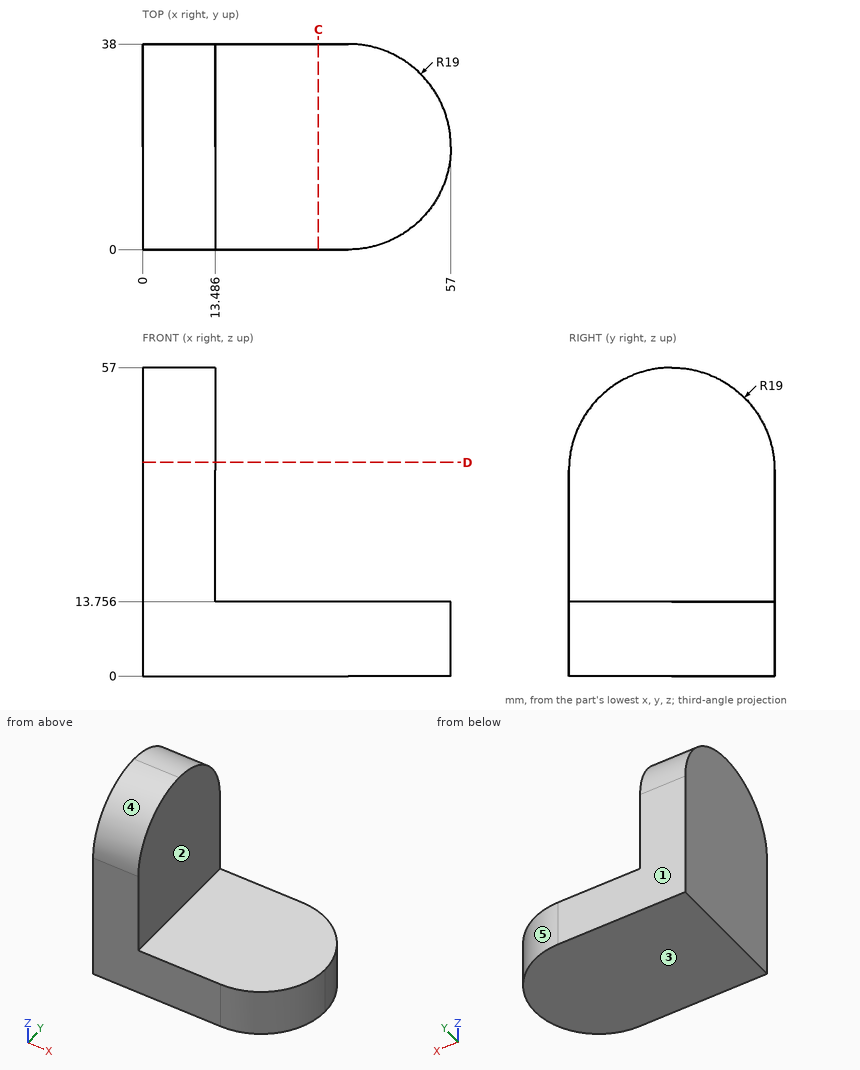
Geometry check sheet. Reference: drawing and pictorial views, mm from the part's lowest x, y, z. A direction names the side the tool comes from. Coordinates: 2 decimals unless noted, no trailing zeros. Order: outer loops, then holes, each group sorted by start corner. A loop starts at its lowest first (then second) coordinate and runs counter-clockwise, first axis right, second up. Notation, with made-up numbers: M 33,67.25 L 80,67.25 A26 cw 80,97.25 Z; hole C -11,57 d7. An arc over 180 degrees is marked long. Write each question's results on one line, items separated by ' | '. Start each with the question number.
1. Mould release check, pull along Z, two halves, no side actions. Record for the marked faces 3, 4 and 5: +Z half, -Z half, draft (parallel to the pull), parting line (faces both ways), or undercut.
2. Material ranges on probe 1 along X at (y, z) = (25, 49) (1 decimal); probe 2 along Z at (x, y) = (47, 27) (1 decimal); probe 3 along X at (y, z) = (18.5, 9), recorded low to high.
3. Go/stop test with flat-tipped pins: P1, Ø10, axis at y = 17.5, z = 29.5, coming from the +X side; P2, Ø3, axis at y = 25.5, z = 41, coming from the -X side; P3, Ø12, axis at x = 44.5, z = 12.5, coming from the +Y side; P4, Ø10, axis at x = 30.5, y = 5.5, coming from the +Z side. Record where each tip stops, or that it passes through.
4. Cross-section at D-D on z = 39.5. Record the cut outline in (x, y) (1 decimal), and give its area (3 significant figures).
5. Access from +Z, -Z, +X, -X, +Y, -Y to the whole of each face (thin tool, end or side, straight path). Record for the marked faces 1 and 2.
6. Cross-section at C-C on x = 32.5. Record the cut outline in (y, z) (1 decimal).
Checks:
1) face 3: -Z half | face 4: +Z half | face 5: draft
2) probe 1: x = 0 to 13.5 | probe 2: z = 0 to 13.8 | probe 3: x = 0 to 56.99
3) P1: stops at x = 13.49 | P2: stops at x = 0 | P3: stops at y = 37.99 | P4: stops at z = 13.76
4) outline: M 0,0.1 L 13.5,0.1 L 13.5,37.9 L 0,37.9 Z | area: 511 mm²
5) face 1: +Z, -Z, +X, -X, +Y | face 2: +Z, +X, +Y, -Y
6) outline: M 0,0 L 38,0 L 38,13.8 L 0,13.8 Z
